Here's how the part is built. I have some questions about the finished solid (model axes, mm). A direction names the side the tool comes from. Give positions to 0.01 mm unless a question says otherwise; leave off trailing zeros. Write each loop counter-clockwise with the first axis right and the second up, starting at its lowest first coordinate (ties: lowest second). Pieces come first, ordered by that corner, then holes. Notation, with made-up numbers: (-19.75, -9.75) - (-11.75, -9.75) arc R22 ccw to (-11.75, 22.25) - close; hole circle Ø9 at (59.5, 59.5). An arc over 180 degrees is marked (long way). Use a Markdown table: item, result.
```python
from build123d import *

# Parameters (mm, degrees)
SKETCH_R           = 32
SKETCH_R_2         = 14
PAD_DEPTH          = 1
SKETCH001_R        = 24.75
SKETCH001_R_2      = 23.75
PAD001_DEPTH       = 1.5
POCKET_DEPTH       = 182.089376
POLARPATTERN_COUNT = 8


with BuildPart() as part:
    # Sketch → Pad (new body)
    with BuildSketch(Plane.XY):
        Circle(SKETCH_R)
        Circle(SKETCH_R_2, mode=Mode.SUBTRACT)
    extrude(amount=PAD_DEPTH)

    # Sketch001 (on Face4 of Pad) → Pad001 (join)
    with BuildSketch(Plane.XY.offset(1)):
        Circle(SKETCH001_R)
        Circle(SKETCH001_R_2, mode=Mode.SUBTRACT)
    extrude(amount=PAD001_DEPTH)

    # Sketch002 (on Face6 of Pad001) → Pocket (cut, through all)
    with BuildSketch(Plane.XY.offset(1)):
        with BuildLine():
            ThreePointArc((9.754466, 12.045762), (5.174006, 14.610943), (0, 15.5))
            ThreePointArc((0, 16.5), (-0.5, 16), (0, 15.5))
            ThreePointArc((10.383786, 12.822908), (5.507813, 15.553585), (0, 16.5))
            ThreePointArc((9.754466, 12.045762), (10.457699, 12.119675), (10.383786, 12.822908))
        make_face()
        with BuildLine():
            ThreePointArc((12.271748, 15.154346), (6.509234, 18.381509), (0, 19.5))
            ThreePointArc((0, 20.5), (-0.5, 20), (0, 19.5))
            ThreePointArc((12.901068, 15.931492), (6.843041, 19.324151), (0, 20.5))
            ThreePointArc((12.271748, 15.154346), (12.974981, 15.228259), (12.901068, 15.931492))
        make_face()
    pocket = extrude(amount=-POCKET_DEPTH, mode=Mode.SUBTRACT)

    # PolarPattern: Pocket ×8 about axis
    polarpattern_axis = Axis((0, 0, 1), (0, 0, 1))
    for i in range(1, POLARPATTERN_COUNT):
        add(pocket.rotate(polarpattern_axis, i * 360 / POLARPATTERN_COUNT), mode=Mode.SUBTRACT)


solid = part.part
```
Item 1: If we section it at D-D, the plane y = 23: Write out the boundary of the cut face in (x, z), plus the area to 3 significant figures.
Values:
| item | result |
|---|---|
| outline | (-22.25, 0) - (22.25, 0) - (22.25, 1) - (9.14, 1) - (9.14, 2.5) - (5.92, 2.5) - (5.92, 1) - (-5.92, 1) - (-5.92, 2.5) - (-9.14, 2.5) - (-9.14, 1) - (-22.25, 1) - close |
| area | 54.2 mm2 |
Item 2: Will these pins go through, and if not, where does the flat tip stop? pin 1 Ø19 at (x, y) = (10.5, -8.5) entering from +Z; pin 2 Ø1.5 at (y, z) = (14.5, 1.5) entering from -X.
Values:
| item | result |
|---|---|
| pin 1 | stops at z = 1 |
| pin 2 | stops at x = -28.8 |
Item 3: I need wall thicknesses on line 1 along X through (y, z) = (4, 0.9); line 2 along Y through (x, z) = (0, 1.55); line 3 along X through (y, z) = (-6.5, 0.6). Which ranges of each line are inside material? Lowest first, please. Write a range as [from, to].
Values:
| item | result |
|---|---|
| line 1 | x = [-31.75, -20.11], [-19.09, -16.01], [-14.97, -13.42], [13.42, 14.97], [16.01, 19.09], [20.11, 31.75] |
| line 2 | y = [-24.75, -23.75], [23.75, 24.75] |
| line 3 | x = [-31.33, -19.44], [-18.38, -15.17], [-14.07, -12.4], [12.4, 14.07], [15.17, 18.38], [19.44, 31.33] |
Item 4: If we section it at A-A, the plane y = 6: Count the separate pieces of the cut face and the enclosed holes in it, plus the area to 3 significant figures.
Values:
| item | result |
|---|---|
| separate pieces | 6 |
| enclosed holes | 0 |
| area | 36.4 mm2 |
Item 5: Thinking about a two-plate mould opening in X: for faces 1 (the cylindrical face through (-3.22, 24.54, 1.74)), 2 (the cylindrical face through (8.31, -17.64, 0.51)), 3 (the cylindrical face through (-6.6, -18.35, 0.51)), 4 (the flat face through (-9.3, 22.1, 2.5)), which applies, +X half, -X half, draft (parallel to the pull), parting line (faces both ways), or undercut?
Values:
| item | result |
|---|---|
| face 1 | parting line |
| face 2 | undercut |
| face 3 | undercut |
| face 4 | draft |
Item 6: If we section it at B-B, the plane z = 1.65: Write out the boundary of the cut face in (x, y), plus the area to 3 significant figures.
Values:
| item | result |
|---|---|
| outline | circle Ø49.5 at (0, 0); hole circle Ø47.5 at (0, 0) |
| area | 152 mm2 |
Item 7: If we section it at C-C, the plane x = -22.5: Write out the boundary of the cut face in (y, z), plus the area to 3 significant figures.
Values:
| item | result |
|---|---|
| outline | (-22.75, 0) - (22.75, 0) - (22.75, 1) - (10.31, 1) - (10.31, 2.5) - (7.6, 2.5) - (7.6, 1) - (-7.6, 1) - (-7.6, 2.5) - (-10.31, 2.5) - (-10.31, 1) - (-22.75, 1) - close |
| area | 53.6 mm2 |
Item 8: For faces 5 (the flat face through (10.2, -10.2, 1)), 6 (the cylindrical face through (15.527, -5.582, 0.507)), 7 (the flat face through (13.8, -6.7, 0)), which set-ups out of +Z, -Z, +X, -X, +Y, -Y let a thin tool reach every point of the face, with its end or its side?
Values:
| item | result |
|---|---|
| face 5 | +Z |
| face 6 | +Z, -Z |
| face 7 | -Z, +X, -X, +Y, -Y |
